```python
from build123d import *

# Parameters (mm, degrees)
BOSS_EXTRUDE1_DEPTH     = 20
FILLET1_R               = 10
SHELL1_T                = -3
SKETCH2_W               = 3
SKETCH2_H               = 40
BOSS_EXTRUDE2_DEPTH     = 20
SKETCH3_W               = 103
SKETCH3_H               = 40
BOSS_EXTRUDE3_DEPTH     = 3
SKETCH4_R               = 1.5
CUT_EXTRUDE1_DEPTH      = 3
LPATTERN1_COUNT         = 5
LPATTERN1_PITCH         = 10
LPATTERN1_COL_COUNT     = 5
LPATTERN1_COL_PITCH     = 10
MIRROR1_COPY_1_SKETCH_R = 1.5
MIRROR1_COPY_1_DEPTH    = 3
MIRROR1_COPY_2_SKETCH_R = 1.5
MIRROR1_COPY_2_DEPTH    = 3
MIRROR1_COPY_3_SKETCH_R = 1.5
MIRROR1_COPY_3_DEPTH    = 3
MIRROR1_COPY_4_SKETCH_R = 1.5
MIRROR1_COPY_4_DEPTH    = 3
MIRROR1_COPY_5_SKETCH_R = 1.5
MIRROR1_COPY_5_DEPTH    = 3
MIRROR1_COPY_6_SKETCH_R = 1.5
MIRROR1_COPY_6_DEPTH    = 3
MIRROR1_COPY_7_SKETCH_R = 1.5
MIRROR1_COPY_7_DEPTH    = 3
MIRROR1_COPY_8_SKETCH_R = 1.5
MIRROR1_COPY_8_DEPTH    = 3


with BuildPart() as part:
    # Sketch1 → Boss-Extrude1 (new body)
    with BuildSketch(Plane(origin=(0, 0, 0), x_dir=(1, 0, 0), z_dir=(0, 1, 0))):
        with BuildLine():
            Line((115.839038172, -85), (130, -85))
            ThreePointArc((130, -85), (144.142135624, -79.142135624), (150, -65))
            Line((150, -65), (150, 65))
            ThreePointArc((150, 65), (144.142135624, 79.142135624), (130, 85))
            Line((130, 85), (-130, 85))
            ThreePointArc((-130, 85), (-144.142135624, 79.142135624), (-150, 65))
            Line((-150, 65), (-150, -65))
            ThreePointArc((-150, -65), (-144.142135624, -79.142135624), (-130, -85))
            Line((-130, -85), (-115.839038172, -85))
            ThreePointArc((-115.839038172, -85), (-110.364546156, -84.236162226), (-105.30821652, -82.002993717))
            ThreePointArc((-105.30821652, -82.002993717), (0, -52.032930885), (105.30821652, -82.002993717))
            ThreePointArc((105.30821652, -82.002993717), (110.364546156, -84.236162226), (115.839038172, -85))
        make_face()
    extrude(amount=BOSS_EXTRUDE1_DEPTH)

    # Fillet1
    fillet1_edges = [part.edges().sort_by_distance(p)[0] for p in [
        (-150, 0, 0),
        (-144.142135624, 0, -79.142135624),
        (0, 0, -85),
        (144.142135624, 0, -79.142135624),
        (150, 0, 0),
        (144.142135624, 0, 79.142135624),
        (122.919519086, 0, 85),
        (110.364546156, 0, 84.236162226),
        (0, 0, 52.032930885),
        (-110.364546156, 0, 84.236162226),
        (-122.919519086, 0, 85),
        (-144.142135624, 0, 79.142135624),
    ]]
    fillet(fillet1_edges, radius=FILLET1_R)

    # Shell1
    shell1_openings = [part.faces().sort_by_distance(p)[0] for p in [
        (0, 20, 25.458771278),
    ]]
    offset(amount=SHELL1_T, openings=shell1_openings, kind=Kind.INTERSECTION)

    # Sketch2 → Boss-Extrude2 (add)
    with BuildSketch(Plane.XZ):
        with Locations((50, 0)):
            Rectangle(SKETCH2_W, SKETCH2_H)
        with Locations((-50, 0)):
            Rectangle(SKETCH2_W, SKETCH2_H)
    extrude(amount=BOSS_EXTRUDE2_DEPTH)

    # Sketch3 → Boss-Extrude3 (add)
    with BuildSketch(Plane.XZ.offset(20)):
        Rectangle(SKETCH3_W, SKETCH3_H)
    extrude(amount=BOSS_EXTRUDE3_DEPTH)

    # Sketch4 → Cut-Extrude1 (cut)
    with BuildSketch(Plane.XZ.offset(23)):
        with Locations((0, 15)):
            Circle(SKETCH4_R)
    cut_extrude1 = extrude(amount=-CUT_EXTRUDE1_DEPTH, mode=Mode.SUBTRACT)

    # LPattern1: Cut-Extrude1 ×5
    with Locations(*[(i * LPATTERN1_PITCH, 0, 0) for i in range(1, LPATTERN1_COUNT)]):
        add(cut_extrude1, mode=Mode.SUBTRACT)

    # LPattern1 col: Cut-Extrude1 ×5
    with Locations(*[(-i * LPATTERN1_COL_PITCH, 0, 0) for i in range(1, LPATTERN1_COL_COUNT)]):
        add(cut_extrude1, mode=Mode.SUBTRACT)

    # Mirror1: Cut-Extrude1 across plane
    add(cut_extrude1.mirror(Plane.XY), mode=Mode.SUBTRACT)

    # Mirror1 copy 1 sketch → Mirror1 copy 1 (cut)
    with BuildSketch(Plane(origin=(10, -23, 0), x_dir=(1, 0, 0), z_dir=(0, -1, 0))):
        with Locations((0, -15)):
            Circle(MIRROR1_COPY_1_SKETCH_R)
    extrude(amount=-MIRROR1_COPY_1_DEPTH, mode=Mode.SUBTRACT)

    # Mirror1 copy 2 sketch → Mirror1 copy 2 (cut)
    with BuildSketch(Plane(origin=(20, -23, 0), x_dir=(1, 0, 0), z_dir=(0, -1, 0))):
        with Locations((0, -15)):
            Circle(MIRROR1_COPY_2_SKETCH_R)
    extrude(amount=-MIRROR1_COPY_2_DEPTH, mode=Mode.SUBTRACT)

    # Mirror1 copy 3 sketch → Mirror1 copy 3 (cut)
    with BuildSketch(Plane(origin=(30, -23, 0), x_dir=(1, 0, 0), z_dir=(0, -1, 0))):
        with Locations((0, -15)):
            Circle(MIRROR1_COPY_3_SKETCH_R)
    extrude(amount=-MIRROR1_COPY_3_DEPTH, mode=Mode.SUBTRACT)

    # Mirror1 copy 4 sketch → Mirror1 copy 4 (cut)
    with BuildSketch(Plane(origin=(40, -23, 0), x_dir=(1, 0, 0), z_dir=(0, -1, 0))):
        with Locations((0, -15)):
            Circle(MIRROR1_COPY_4_SKETCH_R)
    extrude(amount=-MIRROR1_COPY_4_DEPTH, mode=Mode.SUBTRACT)

    # Mirror1 copy 5 sketch → Mirror1 copy 5 (cut)
    with BuildSketch(Plane(origin=(-10, -23, 0), x_dir=(1, 0, 0), z_dir=(0, -1, 0))):
        with Locations((0, -15)):
            Circle(MIRROR1_COPY_5_SKETCH_R)
    extrude(amount=-MIRROR1_COPY_5_DEPTH, mode=Mode.SUBTRACT)

    # Mirror1 copy 6 sketch → Mirror1 copy 6 (cut)
    with BuildSketch(Plane(origin=(-20, -23, 0), x_dir=(1, 0, 0), z_dir=(0, -1, 0))):
        with Locations((0, -15)):
            Circle(MIRROR1_COPY_6_SKETCH_R)
    extrude(amount=-MIRROR1_COPY_6_DEPTH, mode=Mode.SUBTRACT)

    # Mirror1 copy 7 sketch → Mirror1 copy 7 (cut)
    with BuildSketch(Plane(origin=(-30, -23, 0), x_dir=(1, 0, 0), z_dir=(0, -1, 0))):
        with Locations((0, -15)):
            Circle(MIRROR1_COPY_7_SKETCH_R)
    extrude(amount=-MIRROR1_COPY_7_DEPTH, mode=Mode.SUBTRACT)

    # Mirror1 copy 8 sketch → Mirror1 copy 8 (cut)
    with BuildSketch(Plane(origin=(-40, -23, 0), x_dir=(1, 0, 0), z_dir=(0, -1, 0))):
        with Locations((0, -15)):
            Circle(MIRROR1_COPY_8_SKETCH_R)
    extrude(amount=-MIRROR1_COPY_8_DEPTH, mode=Mode.SUBTRACT)


solid = part.part
```
Here's how the part is built. I have some questions about the finished solid (model axes, mm). A direction names the side the tool comes from. Give positions to 0.01 mm unless a question says otherwise; leave off trailing zeros. Order: outer loops, then holes, each group sorted by start corner. A loop starts at its lowest first (then second) coordinate and runs counter-clockwise, first axis right, second up. Notation, with made-up numbers: M -2.75,82 L 11.25,82 A18 cw 11.25,97 Z; hole C -33,71 d8. An arc over 180 degrees is marked long. Use a Markdown table: item, result. Add a question column.
1. On a 3-axis mill with a long thin cutter (end or side, diameter ignored), from which of +Z, -Z, +X, -X, +Y, -Y can I reach the whole of each face in a straight line? I mean faces 1 (the cylindrical face through (-110.439, 14.93, 84.257)), 2 (the cylindrical face through (123.02, 3.01, 82.15)), 3 (the flat face through (0, -22, -20)), 4 (the flat face through (2, 15, -82)), 5 (the flat face through (48.5, -10, 0)). Say none if no direction works.
2. Suppose I cut it at A-A (x = -119). List the corners of the cut face in (y, z) for me.
3. Suppose I cut it at D-D (z = -7). List the corners of the cut face in (x, y) for me, and give its area (3 significant figures).
4. Suppose I cut it at B-B (z = 33). List the corners of the cut face in (x, y) for me, and give its area (3 significant figures).
5. For pin 1 Ø16 at (y, z) = (-5.5, -1) entering from +X; pin 2 Ø10 at (y, z) = (1, -62) entering from +X; pin 3 Ø16 at (y, z) = (-8.5, 5.5) entering from -X, each with a flat end and sliding along its axis, tell me the tip position at first contact or that it passes through.
6. Suppose I cut it at C-C (y = 16). List the corners of the cut face in (x, z) for me.
7. I need wall thicknesses on probe 1 along Z at (x, y) = (30, -22); probe 2 along X at (y, z) = (-3, -10); probe 3 along X at (y, z) = (12, -46). Which ranges of each line are inside material? Lowest first, please. Write a range as from..to.
8. If we mould it in two halves opening along Z, with no side actions, what happens to faces 6 (the cylindrical face through (-145, 5.1, 0.9)), 7 (the flat face through (0, -22, 20)), 8 (the cylindrical face through (-143.986, 14.93, -79.297))? For each: +Z half, -Z half, draft (parallel to the pull), parting line (faces both ways), or undercut.
Results list:
| question | item | result |
|---|---|---|
| 1 | face 1 | +Z, +Y, -Y |
| 1 | face 2 | +Z, +X, -X, -Y |
| 1 | face 3 | -Z, +X, -X, -Y |
| 1 | face 4 | +Y |
| 1 | face 5 | +Z, -Z |
| 2 | outline | M 0,-75 A10 ccw 10,-85 L 20,-85 L 20,-82 L 10,-82 A7 cw 3,-75 L 3,75 A7 cw 10,82 L 20,82 L 20,85 L 10,85 A10 ccw 0,75 Z |
| 3 | outline | M -150,10 A10 ccw -140,0 L -51.5,0 L -51.5,-23 L 51.5,-23 L 51.5,0 L 140,0 A10 ccw 150,10 L 150,20 L 147,20 L 147,10 A7 cw 140,3 L -140,3 A7 cw -147,10 L -147,20 L -150,20 Z; hole M -48.5,-20 L 48.5,-20 L 48.5,0 L -48.5,0 Z |
| 3 | area | 1,410 mm² |
| 4 | outline | M -150,10 A10 ccw -140,0 L 140,0 A10 ccw 150,10 L 150,20 L 147,20 L 147,10 A7 cw 140,3 L -140,3 A7 cw -147,10 L -147,20 L -150,20 Z |
| 4 | area | 980 mm² |
| 5 | pin 1 | stops at x = 146.61 |
| 5 | pin 2 | stops at x = 149.17 |
| 5 | pin 3 | stops at x = -51.5 |
| 6 | outline | M -150,-65 A20 ccw -130,-85 L 130,-85 A20 ccw 150,-65 L 150,65 A20 ccw 130,85 L 115.84,85 A20 ccw 105.31,82 A200 cw -105.31,82 A20 ccw -115.84,85 L -130,85 A20 ccw -150,65 Z; hole M -147,-65 A17 ccw -130,-82 L 130,-82 A17 ccw 147,-65 L 147,65 A17 ccw 130,82 L 115.84,82 A17 ccw 106.89,79.45 A203 cw -106.89,79.45 A17 ccw -115.84,82 L -130,82 A17 ccw -147,65 Z |
| 7 | probe 1 | z = -20..-16.5, -13.5..13.5, 16.5..20 |
| 7 | probe 2 | x = -51.5..-48.5, 48.5..51.5 |
| 7 | probe 3 | x = -150..-147, 147..150 |
| 8 | face 6 | undercut |
| 8 | face 7 | +Z half |
| 8 | face 8 | -Z half |
